```python
from build123d import *

# Parameters (mm, degrees)
SKETCH_1_W          = 70
SKETCH_1_H          = 58
EXTRUDE_1_DEPTH     = 4
SKETCH_2_W          = 9
SKETCH_2_H          = 3
EXTRUDE_2_DEPTH     = 60
SKETCH_4_W          = 70
SKETCH_4_H          = 4
EXTRUDE_4_DEPTH     = 9.5
EXTRUDE_START       = -9
EXTRUDE_5_DEPTH     = 4
SKETCH_5_R          = 50
EXTRUDE_6_DEPTH     = 4
SKETCH_6_R          = 32.5
EXTRUDE_7_DEPTH     = 6
SKETCH_7_R          = 20
CUT_EXTRUDE_1_DEPTH = 6
SKETCH_8_R          = 2.7
CUT_EXTRUDE_2_DEPTH = 10
SKETCH_9_R          = 2.7
CUT_EXTRUDE_3_DEPTH = 10
SKETCH_11_R         = 11.2
SKETCH_11_R_2       = 1.7
EXTRUDE_8_DEPTH     = 3
SKETCH_13_R         = 1.65
SKETCH_13_R_2       = 1.7
CUT_EXTRUDE_4_DEPTH = 10
EXTRUDE_9_DEPTH     = 5


with BuildPart() as part:
    # 草图1 → 凸台-拉伸1 (new body)
    with BuildSketch(Plane.XY):
        Rectangle(SKETCH_1_W, SKETCH_1_H)
    extrude(amount=EXTRUDE_1_DEPTH)

    # 草图2 → 凸台-拉伸2 (add)
    with BuildSketch(Plane.XY.offset(4)):
        with Locations((-30.5, 17)):
            Rectangle(SKETCH_2_W, SKETCH_2_H)
        with Locations((30.5, 17)):
            Rectangle(SKETCH_2_W, SKETCH_2_H)
    extrude(amount=EXTRUDE_2_DEPTH)

    # 草图4 → 凸台-拉伸4 (add)
    with BuildSketch(Plane(origin=(0, 29, 0), x_dir=(1, 0, 0), z_dir=(0, 1, 0))):
        with Locations((0, -2)):
            Rectangle(SKETCH_4_W, SKETCH_4_H)
    extrude(amount=EXTRUDE_4_DEPTH)

    # 草图3 → 凸台-拉伸5 (add)
    with BuildSketch(Plane(origin=(35, 0, 0), x_dir=(0, 0, -1), z_dir=(1, 0, 0)).offset(EXTRUDE_START)):
        Polygon((-4, 29), (-40, 18.5), (-40, 15.5), (-40, 5.399002441), (-4, -5.764089994), (-4, -29), (0, -29), (0, 29), align=None)
    extrude_5 = extrude(amount=-EXTRUDE_5_DEPTH)

    # 镜向2: 凸台-拉伸5 across plane
    add(extrude_5.mirror(Plane(origin=(0, 0, 0), x_dir=(0, 0, 1), z_dir=(1, 0, 0))))

    # 草图5 → 凸台-拉伸6 (add)
    with BuildSketch(Plane(origin=(0, 0, 0), x_dir=(-1, 0, 0), z_dir=(0, 0, -1))):
        with Locations((0, 4.75)):
            Circle(SKETCH_5_R)
    extrude(amount=-EXTRUDE_6_DEPTH)

    # 草图6 → 凸台-拉伸7 (add)
    with BuildSketch(Plane(origin=(0, 0, 0), x_dir=(-1, 0, 0), z_dir=(0, 0, -1))):
        with Locations((0, 4.75)):
            Circle(SKETCH_6_R)
    extrude(amount=EXTRUDE_7_DEPTH)

    # 草图7 → 切除-拉伸1 (cut)
    with BuildSketch(Plane(origin=(0, 0, -6), x_dir=(-1, 0, 0), z_dir=(0, 0, -1))):
        with Locations((0, 4.75)):
            Circle(SKETCH_7_R)
    extrude(amount=-CUT_EXTRUDE_1_DEPTH, mode=Mode.SUBTRACT)

    # 草图8 → 切除-拉伸2 (cut)
    with BuildSketch(Plane(origin=(0, 0, -6), x_dir=(-1, 0, 0), z_dir=(0, 0, -1))):
        with Locations((0, -20.247950199)):
            Circle(SKETCH_8_R)
        with Locations((0, 29.747950199)):
            Circle(SKETCH_8_R)
    extrude(amount=-CUT_EXTRUDE_2_DEPTH, mode=Mode.SUBTRACT)

    # 草图9 → 切除-拉伸3 (cut)
    with BuildSketch(Plane(origin=(0, 0, 0), x_dir=(-1, 0, 0), z_dir=(0, 0, -1))):
        with Locations((-16, 4.75)):
            Circle(SKETCH_9_R)
        with Locations((16, 4.75)):
            Circle(SKETCH_9_R)
    extrude(amount=-CUT_EXTRUDE_3_DEPTH, mode=Mode.SUBTRACT)

    # 草图11 → 凸台-拉伸8 (add)
    with BuildSketch(Plane(origin=(0, 10, 0), x_dir=(1, 0, 0), z_dir=(0, 1, 0))):
        Polygon((-17.5, -4), (17.5, -4), (22, -4), (22, -40), (17.5, -40), (-17.5, -40), (-22, -40), (-22, -4), align=None)
        with Locations(Location((0, -22.5, 0), (0, 0, 180))):
            Circle(SKETCH_11_R, mode=Mode.SUBTRACT)
        with Locations(Location((-13, -9.5, 0), (0, 0, 180))):
            Circle(SKETCH_11_R_2, mode=Mode.SUBTRACT)
        with Locations(Location((13, -9.5, 0), (0, 0, 180))):
            Circle(SKETCH_11_R_2, mode=Mode.SUBTRACT)
        with Locations(Location((13, -35.5, 0), (0, 0, 180))):
            Circle(SKETCH_11_R_2, mode=Mode.SUBTRACT)
        with Locations(Location((-13, -35.5, 0), (0, 0, 180))):
            Circle(SKETCH_11_R_2, mode=Mode.SUBTRACT)
    extrude(amount=EXTRUDE_8_DEPTH)

    # 草图13 → 切除-拉伸4 (cut)
    with BuildSketch(Plane.XZ.offset(-15.5)):
        with Locations(Location((30.5, 11.8, 0), (0, 0, 270))):
            Circle(SKETCH_13_R)
        with Locations(Location((30.5, 31.8, 0), (0, 0, 270))):
            Circle(SKETCH_13_R)
        with Locations(Location((30.5, 51.8, 0), (0, 0, 270))):
            Circle(SKETCH_13_R)
        with Locations(Location((-30.5, 12.2, 0), (0, 0, 270))):
            Circle(SKETCH_13_R_2)
        with Locations(Location((-30.5, 32.2, 0), (0, 0, 270))):
            Circle(SKETCH_13_R_2)
        with Locations(Location((-30.5, 52.2, 0), (0, 0, 270))):
            Circle(SKETCH_13_R_2)
    extrude(amount=-CUT_EXTRUDE_4_DEPTH, mode=Mode.SUBTRACT)

    # 草图14 → 凸台-拉伸9 (add)
    with BuildSketch(Plane.XY.offset(4)):
        Polygon((26, 9), (35, 9), (35, 15.5), (35, 18.5), (37, 18.5), (37, 7), (26, 7), align=None)
    extrude_9 = extrude(amount=EXTRUDE_9_DEPTH)

    # 镜向3: 凸台-拉伸9 across plane
    add(extrude_9.mirror(Plane(origin=(0, 0, 0), x_dir=(0, 0, 1), z_dir=(1, 0, 0))))


solid = part.part
```
The listing builds one solid part. Answer for the finished solid, in the listing's coordinates (mm). A direction names the side the tool comes from. Give positions to 0.01 mm unless a question says otherwise; leave off trailing zeros. Order: outer loops, then holes, each group sorted by start corner. A loop starts at its lowest first (then second) coordinate and runs counter-clockwise, first axis right, second up. Notation, with made-up numbers: (22.5, 59) -> (67.5, 59) arc R32 cw to (67.5, 90) -> close; hole circle Ø9 at (-2, -36.5). An arc over 180 degrees is marked (long way). Answer as a JSON object with one key per item and string values. Group by question number.
Item 1: Flat-ended cylindrical pins translate along their axes: pin 1 (5.5 mm diameter, centred on x = 13, z = 9.5, fed in from +Y); pin 2 (0.9 mm diameter, centred on y = 17, z = 56.5, fed in from -X); pin 3 (3 mm diameter, centred on x = -7.5, y = 26, fed in from +Z). Find the tip coordinate at first contact, or state that the pin passes through.
Item 2: The part is cut by section D-D on x = -17. Write down the section's boundary in (y, z), and give its area (3 significant figures).
Item 3: The part is cut by section A-A on z = 43. Write down the section's boundary in (x, y).
Item 4: The part is cut by section C-C on z = 31.8. Give the number of separate pieces and of enclosed holes in the cut face, and give its area (3 significant figures).
Item 5: Consider L1, parallel to Y at x = 0, z = -1.5; L2, parallel to Z at x = -13, y = 11; L3, parallel to Z at x = -30, y = 16. Determine where each line is inside the solid, lowest interval first. Write a range as from..to.
Item 6: A tool of negligible diameter and unlimited length cuts with its end or side. For faces 5 (the flat face through (35, 17, 37)), 6 (the flat face through (0, 12, 40)), 7 (the flat face through (-22, 19, 18)), 8 (the flat face through (-35, 17, 37)), 9 (the flat face through (-32, 15.5, 34)), from which of +Z, -Z, +X, -X, +Y, -Y can it reach the whole face along a straight path? Write none if from no direction.
Item 7: Determine the mould class of faces 1 (the flat face through (31, 12, 4)), 2 (the flat face through (32, 7, 6)), 3 (the flat face through (30, 17, 64)), 4 (the flat face through (30, 9, 6)) for opening direction Y: pulls with the +Y half, pulls with the -Y half, needs draft (parallel to the pull), parting line crosses it, or undercut.
Item 8: The part is cut by section B-B on x = 0. Write down the section's boundary in (y, z), and give its area (3 significant figures).
Result set:
{
 "1": {"pin 1": "y = 13", "pin 2": "x = -35", "pin 3": "z = 4"},
 "2": {"outline": "(-42.27, 0) -> (-22.95, 0) -> (-22.95, -6) -> (-5.79, -6) -> (-5.79, 0) -> (2.24, 0) -> (2.24, 4) -> (-42.27, 4) -> close; (7.26, 0) -> (15.29, 0) -> (15.29, -6) -> (32.45, -6) -> (32.45, 0) -> (51.77, 0) -> (51.77, 4) -> (13, 4) -> (13, 40) -> (10, 40) -> (10, 4) -> (7.26, 4) -> close", "area": "670 mm²"},
 "3": {"outline": "(-35, 15.5) -> (-26, 15.5) -> (-26, 18.5) -> (-35, 18.5) -> close; (26, 15.5) -> (35, 15.5) -> (35, 18.5) -> (26, 18.5) -> close"},
 "4": {"separate pieces": "4", "enclosed holes": "0", "area": "273 mm²"},
 "5": {"L1": "-27.75..-22.95, -17.55..-15.25, 24.75..27.05, 32.45..37.25", "L2": "0..7.8, 11.2..33.8, 37.2..40", "L3": "-6..10.58, 13.82..30.58, 33.82..50.58, 53.82..64"},
 "6": {"face 5": "+Z, +X, +Y, -Y", "face 6": "+Z, +Y, -Y", "face 7": "+Z, +Y", "face 8": "+Z, -X, +Y, -Y", "face 9": "+Z"},
 "7": {"face 1": "undercut", "face 2": "pulls with the -Y half", "face 3": "needs draft", "face 4": "undercut"},
 "8": {"outline": "(-45.25, 0) -> (-27.75, 0) -> (-27.75, -6) -> (-22.95, -6) -> (-22.95, 4) -> (-45.25, 4) -> close; (-17.55, -6) -> (-15.25, -6) -> (-15.25, 0) -> (24.75, 0) -> (24.75, -6) -> (27.05, -6) -> (27.05, 4) -> (13, 4) -> (13, 11.3) -> (10, 11.3) -> (10, 4) -> (-17.55, 4) -> close; (10, 33.7) -> (13, 33.7) -> (13, 40) -> (10, 40) -> close; (32.45, -6) -> (37.25, -6) -> (37.25, 0) -> (54.75, 0) -> (54.75, 4) -> (32.45, 4) -> close", "area": "483 mm²"}
}
